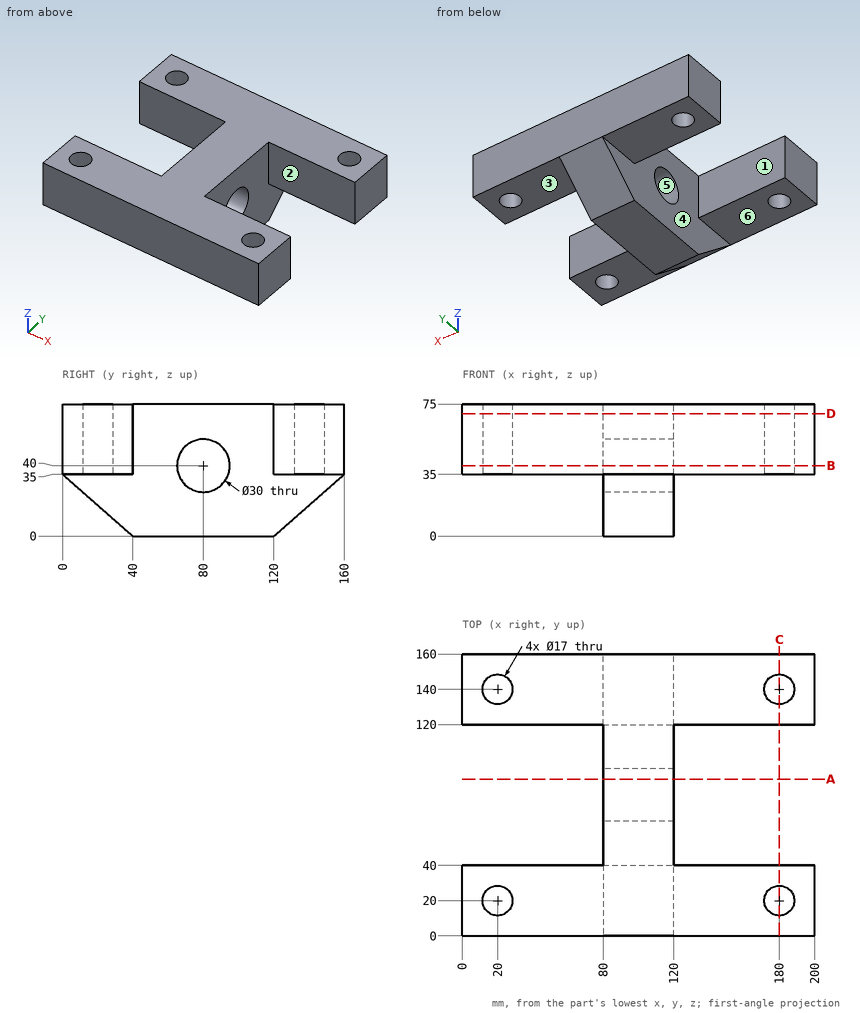
The drawing under review shows one solid part. Ordinate dimensions are in mm from its lowest x, y, z. A direction names the side the tool comes from. Give positions to 0.01 mm unless a question says otherwise; leave off trailing zeros. Write each loop counter-clockwise with the first axis right and the second up, starting at its lowest first coordinate (ties: lowest second). Pieces come first, ordered by that corner, then holes. Notation, with made-up numbers: (63.5, 68.5) -> (113.5, 68.5) arc R30 cw to (113.5, 107.5) -> close; hole circle Ø6 at (-24, 38.5). An arc over 180 degrees is marked (long way). Put each result on its own line as item: value.
(1) The part is to be moulded in two halves that separate along Z. For the marked faces 4, 5 and 6, say which applies: pulls with the +Z half, pulls with the -Z half, needs draft (parallel to the pull), parting line crosses it, or undercut.
Results are:
face 4: needs draft
face 5: undercut
face 6: pulls with the -Z half
(2) For pin 1 Ø1.5 at (x, y) = (162.5, 23.5) entering from -Z; pin 2 Ø12 at (y, z) = (75.5, 27.5) entering from +X, all flat-tipped, find the tip position at first contact; note any pin that passes through.
Results are:
pin 1: z = 35
pin 2: x = 120
(3) Tool access review of the marked faces 1, 2 and 3: name each direction out of +Z, -Z, +X, -X, +Y, -Y from which nothing blocks a thin tool from reaching the whole face with its end or side.
Results are:
face 1: +Z, -Z, -X
face 2: +Z, -Z, +X
face 3: -Z, +X, +Y, -Y
(4) To check wall thickness, follow probe 1 along Y at (x, z) = (180, 43); probe 2 along Y at (x, z) = (125, 64); probe 3 along X at (y, z) = (27.5, 49.5). State the ranges of each line that lie inside material, in increasing order. Write a range as from..to.
Results are:
probe 1: 0..11.5, 28.5..40, 120..131.5, 148.5..160
probe 2: 0..40, 120..160
probe 3: 0..16, 24..176, 184..200
(5) We need section A-A, the plane y = 89. Give the boundary of the cut face in (x, z).
Results are:
outline: (80, 0) -> (120, 0) -> (120, 28) -> (80, 28) -> close; (80, 52) -> (120, 52) -> (120, 75) -> (80, 75) -> close
(6) We need section C-C, the plane x = 180. Give the boundary of the cut face in (y, z), and give its area (3 significant figures).
Results are:
outline: (0, 35) -> (11.5, 35) -> (11.5, 75) -> (0, 75) -> close; (28.5, 35) -> (40, 35) -> (40, 75) -> (28.5, 75) -> close; (120, 35) -> (131.5, 35) -> (131.5, 75) -> (120, 75) -> close; (148.5, 35) -> (160, 35) -> (160, 75) -> (148.5, 75) -> close
area: 1,840 mm²
(7) We need section D-D, the plane z = 69.5. Give the boundary of the cut face in (x, y), and give its area (3 significant figures).
Results are:
outline: (0, 0) -> (200, 0) -> (200, 40) -> (120, 40) -> (120, 120) -> (200, 120) -> (200, 160) -> (0, 160) -> (0, 120) -> (80, 120) -> (80, 40) -> (0, 40) -> close; hole circle Ø17 at (20, 20); hole circle Ø17 at (20, 140); hole circle Ø17 at (180, 20); hole circle Ø17 at (180, 140)
area: 18,300 mm²
(8) We need section B-B, the plane z = 40. Give the boundary of the cut face in (x, y), and give its area (3 significant figures).
Results are:
outline: (0, 0) -> (200, 0) -> (200, 40) -> (120, 40) -> (120, 65) -> (80, 65) -> (80, 40) -> (0, 40) -> close; (0, 120) -> (80, 120) -> (80, 95) -> (120, 95) -> (120, 120) -> (200, 120) -> (200, 160) -> (0, 160) -> close; hole circle Ø17 at (20, 20); hole circle Ø17 at (20, 140); hole circle Ø17 at (180, 20); hole circle Ø17 at (180, 140)
area: 17,100 mm²
